Geometry check sheet. Reference: the model listing, model coordinates, mm. Round coordinates to 2 decimals unless told otherwise and drop trailing zeros. Write each loop counter-clockwise with the first axis right and the second up, starting at its lowest first coordinate (ties: lowest second). Pieces come first, ordered by that corner, then holes. Notation, with made-up numbers: M 73.25,20 L 78.25,20 A31 ccw 78.25,45 Z; hole C -15,72.5 d1. An arc over 180 degrees is marked long. One line per item, written item: value. Start each with the question number.
1. Scan lines: probe 1 along Z at (x, y) = (0.5, 0); probe 2 along X at (y, z) = (0.1, 0.5); probe 3 along X at (y, z) = (-0.9, 2.75). Record each from-to range of solid material in increasing order. Write a range as [from, to].
2. Release check for a two-part mould opening along X. For faces 1 (the cylindrical face through (-3.32, -0.01, -0.74)), 2 (the flat face through (-5.22, 0.02, 2.96)), 3 (the flat face through (0, 0, 6)), 4 (the flat face through (5.172, 0.016, 3.042)) record: pulls with the +X half, pulls with the -X half, needs draft (parallel to the pull), parting line crosses it, or undercut.
3. Section check B-B (y = -0.5). Record the boundary of the cut face in (x, z).
4. Section check C-C (y = 0.9). Record the boundary of the cut face in (x, z).
5. Section check A-A (x = 0). Record the boundary of the cut face in (y, z), and give its area (3 significant figures).
from build123d import *

# Parameters (mm, degrees)
SKETCH1_R           = 3.4
BOSS_EXTRUDE1_DEPTH = 1.2
CHAMFER1_SIZE       = 0.5


with BuildPart() as part:
    # Sketch1 → Boss-Extrude1 (new, symmetric)
    with BuildSketch(Plane(origin=(0, 0, 0), x_dir=(1, 0, 0), z_dir=(0, 1, 0))):
        Polygon((3.464101615, 6), (-3.464101615, 6), (-6.92820323, 0), (-3.464101615, -6), (3.464101615, -6), (6.92820323, 0), align=None)
        with Locations(Location((0, 0, 0), (0, 0, 270))):
            Circle(SKETCH1_R, mode=Mode.SUBTRACT)
    extrude(amount=BOSS_EXTRUDE1_DEPTH, both=True)

    # Chamfer1
    chamfer1_edges = [part.edges().sort_by_distance(p)[0] for p in [
        (0, -1.2, -3.4),
        (0, 1.2, -3.4),
    ]]
    chamfer(chamfer1_edges, length=CHAMFER1_SIZE)

    # Sketch3 → Cut-Revolve1 (revolve, cut)
    with BuildSketch(Plane.XY, mode=Mode.PRIVATE) as cut_revolve1_sk:
        Polygon((6.92820323, 1.2), (6.92820323, 0.7), (5.92820323, 1.2), align=None)
        Polygon((5.92820323, -1.2), (6.92820323, -1.2), (6.92820323, -0.7), align=None)
    revolve(cut_revolve1_sk.sketch.rotate(Axis((0, 0, 0), (0, 1, 0)), 300.000000007), axis=Axis((0, 0, 0), (0, 1, 0)), mode=Mode.SUBTRACT)


solid = part.part
Result sheet:
1. probe 1: z = [-6, -3.36], [3.36, 6]
1. probe 2: x = [-6.64, -3.36], [3.36, 6.64]
1. probe 3: x = [-5.34, -2.32], [2.32, 5.34]
2. face 1: undercut
2. face 2: pulls with the -X half
2. face 3: needs draft
2. face 4: pulls with the +X half
3. outline: M -6.93,0 L -3.46,-6 L 3.46,-6 L 6.93,0 L 3.46,6 L -3.46,6 Z; hole C 0,0 d6.8
4. outline: M -6.48,-0.77 L -3.91,-5.23 A6.53 ccw -2.57,-6 L 2.57,-6 A6.53 ccw 3.91,-5.23 L 6.48,-0.77 A6.53 ccw 6.48,0.77 L 3.91,5.23 A6.53 ccw 2.57,6 L -2.57,6 A6.53 ccw -3.91,5.23 L -6.48,0.77 A6.53 ccw Z; hole C 0,0 d7.2
5. outline: M -1.2,-5.93 L -1.16,-6 L 1.16,-6 L 1.2,-5.93 L 1.2,-3.9 L 0.7,-3.4 L -0.7,-3.4 L -1.2,-3.9 Z; M -1.2,3.9 L -0.7,3.4 L 0.7,3.4 L 1.2,3.9 L 1.2,5.93 L 1.16,6 L -1.16,6 L -1.2,5.93 Z
5. area: 12.0 mm2
